from build123d import *

# Parameters (mm, degrees)
F0_R     = 1.5875
F1_DEPTH = 25.4


with BuildPart() as f1:
    # F0 (on Front) → F1 (new body)
    with BuildSketch(Plane.XZ):
        with BuildLine():
            ThreePointArc((-44.9749847751, 74.0057436376), (-42.239710519, 67.1728704693), (-35.4511886835, 64.3293071628))
            ThreePointArc((-35.4511886835, 64.3293071628), (-28.7159965927, 67.119115072), (-25.9261886835, 73.8543071628))
            ThreePointArc((-25.9261886835, 73.8543071628), (-25.931047818, 74.1585158089), (-25.9456202636, 74.4624140737))
            ThreePointArc((-25.9456202636, 74.4624140737), (-35.6797057153, 83.3765655591), (-44.9749847751, 74.0057436376))
        make_face()
        with BuildLine():
            ThreePointArc((-32.2761886835, 73.8543071628), (-33.2061246532, 71.6092431325), (-35.4511886835, 70.6793071628))
            ThreePointArc((-35.4511886835, 70.6793071628), (-37.6962527138, 76.099371193), (-32.2761886835, 73.8543071628))
        make_face(mode=Mode.SUBTRACT)
        with BuildLine():
            ThreePointArc((-25.9261886835, 73.8543071628), (-28.7159965927, 67.119115072), (-35.4511886835, 64.3293071628))
            Line((-35.4511886835, 64.3293071628), (-35.4511886835, 32.5793071628))
            ThreePointArc((-35.4511886835, 32.5793071628), (-25.8667813668, 29.3595338058), (-20.1702001062, 21.0062849753))
            Line((-20.1702001062, 21.0062849753), (-25.9456202636, 74.4624140737))
            ThreePointArc((-25.9456202636, 74.4624140737), (-25.931047818, 74.1585158089), (-25.9261886835, 73.8543071628))
        make_face()
        with BuildLine():
            Line((-35.4511886835, 32.5793071628), (-35.4511886835, 64.3293071628))
            ThreePointArc((-35.4511886835, 64.3293071628), (-42.239710519, 67.1728704693), (-44.9749847751, 74.0057436376))
            Line((-44.9749847751, 74.0057436376), (-50.7276259168, 21.0224190715))
            ThreePointArc((-50.7276259168, 21.0224190715), (-45.0289127986, 29.3645925377), (-35.4511886835, 32.5793071628))
        make_face()
        with Locations((-40.9250855446, 53.2295071628)):
            Circle(F0_R, mode=Mode.SUBTRACT)
        with BuildLine():
            ThreePointArc((-20.1702001062, 21.0062849753), (-25.8667813668, 29.3595338058), (-35.4511886835, 32.5793071628))
            Line((-35.4511886835, 32.5793071628), (-35.4511886835, 19.8793071628))
            ThreePointArc((-35.4511886835, 19.8793071628), (-33.2061246532, 18.949371193), (-32.2761886835, 16.7043071628))
            ThreePointArc((-32.2761886835, 16.7043071628), (-33.2061246532, 14.4592431325), (-35.4511886835, 13.5293071628))
            Line((-35.4511886835, 13.5293071628), (-35.4511886835, 0.8293071628))
            ThreePointArc((-35.4511886835, 0.8293071628), (-25.1755047485, 4.6036483101), (-19.7859860662, 14.131944055))
            Line((-19.7859860662, 14.131944055), (-19.6039763716, 15.7654318029))
            Line((-19.6039763716, 15.7654318029), (-20.1702001062, 21.0062849753))
        make_face()
        with BuildLine():
            Line((-35.4511886835, 19.8793071628), (-35.4511886835, 32.5793071628))
            ThreePointArc((-35.4511886835, 32.5793071628), (-45.0289127986, 29.3645925377), (-50.7276259168, 21.0224190715))
            Line((-50.7276259168, 21.0224190715), (-51.2984009954, 15.7654318029))
            Line((-51.2984009954, 15.7654318029), (-51.1163913008, 14.131944055))
            ThreePointArc((-51.1163913008, 14.131944055), (-45.7268726185, 4.6036483101), (-35.4511886835, 0.8293071628))
            Line((-35.4511886835, 0.8293071628), (-35.4511886835, 13.5293071628))
            ThreePointArc((-35.4511886835, 13.5293071628), (-38.6261886835, 16.7043071628), (-35.4511886835, 19.8793071628))
        make_face()
        with BuildLine():
            ThreePointArc((-19.7859860662, 14.131944055), (-25.1755047485, 4.6036483101), (-35.4511886835, 0.8293071628))
            Line((-35.4511886835, 0.8293071628), (-35.4511886835, -30.9206928372))
            ThreePointArc((-35.4511886835, -30.9206928372), (-28.7159965927, -33.7105007464), (-25.9261886835, -40.4456928372))
            Line((-25.9261886835, -40.4456928372), (1.0613113165, -40.4456928372))
            ThreePointArc((1.0613113165, -40.4456928372), (3.3861512408, -34.8330327616), (8.9988113165, -32.5081928372))
            Line((8.9988113165, -32.5081928372), (-16.2812915947, -31.605332019))
            ThreePointArc((-16.2812915947, -31.605332019), (-22.0159487809, -28.8548482736), (-23.8988395601, -22.7798029084))
            Line((-23.8988395601, -22.7798029084), (-19.7859860662, 14.131944055))
        make_face()
        with BuildLine():
            Line((-35.4511886835, -30.9206928372), (-35.4511886835, 0.8293071628))
            ThreePointArc((-35.4511886835, 0.8293071628), (-45.7268726185, 4.6036483101), (-51.1163913008, 14.131944055))
            Line((-51.1163913008, 14.131944055), (-44.9176057417, -41.5004786351))
            ThreePointArc((-44.9176057417, -41.5004786351), (-42.5495145328, -34.0943626508), (-35.4511886835, -30.9206928372))
        make_face()
        with BuildLine():
            ThreePointArc((-25.9261886835, -40.4456928372), (-28.7159965927, -33.7105007464), (-35.4511886835, -30.9206928372))
            Line((-35.4511886835, -30.9206928372), (-35.4511886835, -37.2706928372))
            ThreePointArc((-35.4511886835, -37.2706928372), (-33.2061246532, -38.200628807), (-32.2761886835, -40.4456928372))
            Line((-32.2761886835, -40.4456928372), (-25.9261886835, -40.4456928372))
        make_face()
        with BuildLine():
            Line((-35.4511886835, -37.2706928372), (-35.4511886835, -30.9206928372))
            ThreePointArc((-35.4511886835, -30.9206928372), (-42.5495145328, -34.0943626508), (-44.9176057417, -41.5004786351))
            ThreePointArc((-44.9176057417, -41.5004786351), (-41.80251887, -47.5440186865), (-35.4511886835, -49.9706928372))
            Line((-35.4511886835, -49.9706928372), (-34.7716982376, -49.9464253213))
            ThreePointArc((-34.7716982376, -49.9464253213), (-28.4798985771, -46.9362043157), (-25.9261886835, -40.4456928372))
            Line((-25.9261886835, -40.4456928372), (-32.2761886835, -40.4456928372))
            ThreePointArc((-32.2761886835, -40.4456928372), (-37.6962527138, -42.6907568675), (-35.4511886835, -37.2706928372))
        make_face()
        with BuildLine():
            Line((1.0613113165, -40.4456928372), (-25.9261886835, -40.4456928372))
            ThreePointArc((-25.9261886835, -40.4456928372), (-28.4798985771, -46.9362043157), (-34.7716982376, -49.9464253213))
            Line((-34.7716982376, -49.9464253213), (8.9988113165, -48.3831928372))
            ThreePointArc((8.9988113165, -48.3831928372), (3.3861512408, -46.0583529129), (1.0613113165, -40.4456928372))
        make_face()
        with BuildLine():
            ThreePointArc((8.9988113165, -32.5081928372), (3.3861512408, -34.8330327616), (1.0613113165, -40.4456928372))
            ThreePointArc((1.0613113165, -40.4456928372), (3.3861512408, -46.0583529129), (8.9988113165, -48.3831928372))
            ThreePointArc((8.9988113165, -48.3831928372), (14.6114713922, -46.0583529129), (16.9363113165, -40.4456928372))
            ThreePointArc((16.9363113165, -40.4456928372), (14.6114713922, -34.8330327616), (8.9988113165, -32.5081928372))
        make_face()
        with BuildLine():
            ThreePointArc((12.1738113165, -40.4456928372), (8.9988113165, -43.6206928372), (5.8238113165, -40.4456928372))
            ThreePointArc((5.8238113165, -40.4456928372), (8.9988113165, -37.2706928372), (12.1738113165, -40.4456928372))
        make_face(mode=Mode.SUBTRACT)
    extrude(amount=F1_DEPTH)


solid = f1.part
Source: CAD feature listing. Evaluate the final solid. Frame: model axes, mm. Give positions to 0.01 mm unless a question says otherwise; leave off trailing zeros. Order: outer loops, then holes, each group sorted by start corner. A loop starts at its lowest first (then second) coordinate and runs counter-clockwise, first axis right, second up. Notation, with made-up numbers: (-3.75, -4) -> (49.25, -4) arc R18 ccw to (49.25, 7) -> close; hole circle Ø11 at (66, -25). An arc over 180 degrees is marked (long way). Write item = value, one per line.
Item 1: Section query C-C (y = -19.25). State how many separate pieces and enclosed holes the cut face has, then the cut area to 3 significant figures.
Check result:
separate_pieces = 1
enclosed_holes = 5
area = 3,780 mm²
Item 2: Section query B-B (x = -22). Output: boundary loops of the cut face in (y, z), then the cut area to 3 significant figures.
Check result:
outline = (-25.4, -49.49) -> (0, -49.49) -> (0, -28.87) -> (-25.4, -28.87) -> close; (-25.4, -5.74) -> (0, -5.74) -> (0, 37.94) -> (-25.4, 37.94) -> close
area = 1,630 mm²
Item 3: Section query A-A (x = -37). Output: boundary loops of the cut face in (y, z), then the cut area to 3 significant figures.
Check result:
outline = (-25.4, -49.84) -> (0, -49.84) -> (0, -43.22) -> (-25.4, -43.22) -> close; (-25.4, -37.67) -> (0, -37.67) -> (0, 13.93) -> (-25.4, 13.93) -> close; (-25.4, 19.48) -> (0, 19.48) -> (0, 71.08) -> (-25.4, 71.08) -> close; (-25.4, 76.63) -> (0, 76.63) -> (0, 83.25) -> (-25.4, 83.25) -> close
area = 2,960 mm²
Item 4: Contact query for flat-ended pins moving along their axis: pin 1 (8.5 mm diameter, centred on x = 9, z = -40.45, fed in from +Y); pin 2 (5 mm diameter, centred on x = -27, y = -14.5, fed in from -Z); pin 3 (3 mm diameter, centred on y = -16, z = -10.5, fed in from +X); pin 4 (4 mm diameter, centred on x = 9, y = -2.5, fed in from -Z). Output: stop coordinate, or through.
Check result:
pin_1 = 0
pin_2 = -49.76
pin_3 = -22.36
pin_4 = -48.45
Item 5: Ray query, probe 1 along X at (y, z) = (-9, 15); probe 2 along Z at (x, y) = (10, -1.25); probe 3 along X at (y, z) = (-8.5, 77.5). Return the intervals inside material, ascending.
Check result:
probe_1 = -51.21 to -38.13, -32.77 to -19.69
probe_2 = -48.32 to -43.46, -37.43 to -32.57
probe_3 = -44.25 to -26.65
Item 6: Section query D-D (z = -35.5). Output: boundary loops of the cut face in (x, y).
Check result:
outline = (-45.59, -25.4) -> (15.21, -25.4) -> (15.21, 0) -> (-45.59, 0) -> close
Item 7: Mould query, pull axis Z, two halves, no side actions, for faces 1 (the face through (-35.48, -12.52, 83.38)), 2 (the face through (-33, -25.4, 3)), 3 (the face through (9.687, -12.522, -43.545)), 4 (the face through (-41.875, -12.522, -47.479)). Classes: +Z half, -Z half, draft (parallel to the pull), parting line (faces both ways), or undercut.
Check result:
face_1 = +Z half
face_2 = draft
face_3 = undercut
face_4 = -Z half
